Source: CAD feature listing. Evaluate the final solid. Frame: model axes, mm. Coordinates: 2 decimals unless noted, no trailing zeros. Order: outer loops, then holes, each group sorted by start corner. A loop starts at its lowest first (then second) coordinate and runs counter-clockwise, first axis right, second up.
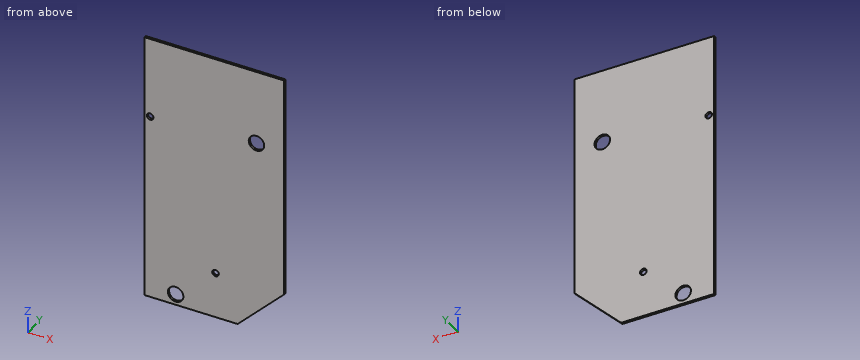
Autodesk Inventor part; units mm, degrees
ref_plane "YZ Plane" through (0, 0, 0) normal (1, 0, 0) x (0, 1, 0)
ref_plane "XZ Plane" through (0, 0, 0) normal (0, 1, 0) x (-1, 0, 0)
ref_plane "XY Plane" through (0, 0, 0) normal (0, 0, 1) x (1, 0, 0)
sketch "Skizze1" plane through (0, 0, 0) normal (0, 1, 0) x (-1, 0, 0)
  line L0 (0, 0) -> (-42, 0)
  line L1 (-63, 21) -> (-63, 123)
  line L2 (-63, 123) -> (0, 123)
  line L3 (0, 123) -> (0, 0)
  line L4 (-42, 0) -> (-63, 21)
  line L5 (-42, 0) -> (-12.3015, 0) construction
  circle A0 centre (-14, 5) radius 3.5
  circle A1 centre (-32, 21) radius 1.5
  circle A2 centre (-2.5, 86) radius 1.5
  circle A3 centre (-50.5, 89) radius 3.5
  dimension "d0" = 63
  dimension "d1" = 102
  dimension "d2" = 135
  dimension "d3" = 42
  dimension "d4" = 7
  dimension "d5" = 3
  dimension "d6" = 3
  dimension "d7" = 7
  dimension "d8" = 2.5
  dimension "d9" = 37
  dimension "d10" = 14
  dimension "d11" = 5
  dimension "d12" = 21
  dimension "d13" = 32
  dimension "d14" = 12.5
  dimension "d15" = 34
extrude "Extrusion1" add sketch "Skizze1" along normal blind 1
properties part number "01_PCBoard"
Q1. Section query C-C on x = 32. Output: boundary loops of the cut face in (y, z), plus the area to 3 significant figures.
Solutions:
outline: (0, 0) - (1, 0) - (1, 19.5) - (0, 19.5) - close; (0, 22.5) - (1, 22.5) - (1, 123) - (0, 123) - close
area: 120 mm2
Q2. Section query D-D on x = 45.5. Output: boundary loops of the cut face in (y, z), plus the area to 4 significant figures.
Solutions:
outline: (0, 3.5) - (1, 3.5) - (1, 123) - (0, 123) - close
area: 119.5 mm2
Q3. Section query A-A on z = 5. Output: boundary loops of the cut face in (x, y), plus the area to 3 significant figures.
Solutions:
outline: (0, 0) - (10.5, 0) - (10.5, 1) - (0, 1) - close; (17.5, 0) - (47, 0) - (47, 1) - (17.5, 1) - close
area: 40.0 mm2
Q4. Section query B-B on y = 0.4. Output: boundary loops of the cut face in (x, z), plus the area to 3 significant figures.
Solutions:
outline: (0, 0) - (42, 0) - (63, 21) - (63, 123) - (0, 123) - close; hole circle Ø3 at (2.5, 86); hole circle Ø7 at (14, 5); hole circle Ø3 at (32, 21); hole circle Ø7 at (50.5, 89)
area: 7,440 mm2
Q5. Material intervals for line 1 along Z through (x, y) = (50.5, 0.3); line 2 along Z through (x, y) = (2.5, 0.4); line 3 along X through (y, z) = (0.45, 86), sorted ascending.
Solutions:
line 1: z = 8.5 to 85.5, 92.5 to 123
line 2: z = 0 to 84.5, 87.5 to 123
line 3: x = 0 to 1, 4 to 48.7, 52.3 to 63
Q6. Pin query (flat end, axial travel): P1, Ø5, axis at x = 32, z = 21, coming from the -Y side. Return the tip coordinate at first contact, or that it passes through.
Solutions:
P1: stops at y = 0
